For this review, take the finished solid that the model builds, in its own axes (mm). A direction names the side the tool comes from. Round coordinates to 2 decimals unless told otherwise and drop trailing zeros. Write each loop counter-clockwise with the first axis right and the second up, starting at its lowest first coordinate (ties: lowest second). Pieces come first, ordered by that corner, then holes. Notation, with made-up numbers: (76, 85) -> (123, 85) arc R37 ccw to (123, 124) -> close; hole circle Ø7 at (11, 48.25). An arc over 180 degrees is marked (long way). Write item = value, one per line. Start each with the question number.
```python
from build123d import *

# Parameters (mm, degrees)
SKETCH_2_R          = 17
CUT_EXTRUDE_1_DEPTH = 10


with BuildPart() as part:
    # Sketch 1 → Revolve 1 (revolve)
    with BuildSketch(Plane.XY, mode=Mode.PRIVATE) as revolve_1_sk:
        Polygon((0, 50), (6.773, 50), (8, 48.773), (8, 10), (12, 10), (15, 9.196152423), (15, 2), (16, 2), (16, 0), (20, 0), (20, -6), (18.5, -6), (18.5, -8), (0, -8), align=None)
    revolve(revolve_1_sk.sketch.rotate(Axis((0, -8, 0), (0, 1, 0)), 270), axis=Axis((0, -8, 0), (0, 1, 0)))

    # Sketch 2 → Cut-Extrude 1 (cut)
    with BuildSketch(Plane(origin=(0, 2, 0), x_dir=(1, 0, 0), z_dir=(0, 1, 0))):
        Circle(SKETCH_2_R)
        Polygon((-12, -6.92820323), (0, -13.856406461), (12, -6.92820323), (12, 6.92820323), (0, 13.856406461), (-12, 6.92820323), align=None, mode=Mode.SUBTRACT)
    extrude(amount=CUT_EXTRUDE_1_DEPTH, mode=Mode.SUBTRACT)


solid = part.part
```
1. Machinability: for faces 1 (the flat face through (6, 2, -11)), 2 (the flat face through (12, 6, 0)), 3 (the flat face through (-6.084, 5.944, 10.344)), 4 (the flat face through (-12, 6, 0)), 5 (the flat face through (-18, -6, 6)), which of the approach directions +Z, -Z, +X, -X, +Y, -Y give a long, thin tool a straight path to every point of the face, cutting with its end or side? Answer none if there is none.
2. Consider section B-B, the plane x = -17. Give the boundary of the cut face in (y, z), then the cut area to 3 significant figures.
3. Clearance check with flat-ended pins moving along their axes: pin 1 Ø1 at (x, z) = (9, -11.5) entering from +Y; pin 2 Ø4 at (x, y) = (-5.5, 39) entering from -Z; pin 3 Ø10 at (x, y) = (3.5, 35) entering from -Z. State where each tip first meets the part, or that it passes through.
4. Consider section A-A, the plane y = 19. Give the boundary of the cut face in (x, z), then the cut area to 3 significant figures.
5. Wall thickness on L1, parallel to Z at x = 0.5, y = 42; L2, parallel to Y at x = 7, z = -12.5; L3, parallel to Y at x = -9.5, z = 14: over which ranges is each line inside the solid? List them lowest first. Write a range as from..to.
6. Draft analysis for pull direction Y (two halves, no side actions). For faces 6 (the flat face through (6.084, 5.944, -10.344)), 7 (the flat face through (0, -8, 0)), 8 (the flat face through (0, 50, 0)), state which applies: +Y half, -Y half, draft (parallel to the pull), parting line (faces both ways), or undercut.
Outcome:
q1.face_1 = +Y
q1.face_2 = +Z, -Z, +X, +Y
q1.face_3 = +Z, -X, +Y
q1.face_4 = +Z, -Z, -X, +Y
q1.face_5 = -Y
q2.outline = (-8, -7.3) -> (-6, -7.3) -> (-6, -10.54) -> (0, -10.54) -> (0, 10.54) -> (-6, 10.54) -> (-6, 7.3) -> (-8, 7.3) -> close
q2.area = 156 mm2
q3.pin_1 = 2
q3.pin_2 = -7.19
q3.pin_3 = -8
q4.outline = circle Ø16 at (0, 0)
q4.area = 201 mm2
q5.L1 = -7.98..7.98
q5.L2 = -8..2
q5.L3 = -8..0
q6.face_6 = draft
q6.face_7 = -Y half
q6.face_8 = +Y half
